from build123d import *

# Parameters (mm, degrees)
SKETCH1_W           = 115
SKETCH1_H           = 50
BOSS_EXTRUDE1_DEPTH = 29
CHAMFER1_SIZE       = 6
FILLET1_R           = 6
SKETCH2_W           = 40
SKETCH2_H           = 32
CUT_EXTRUDE1_DEPTH  = 1
CUT_EXTRUDE2_DEPTH  = 4
SKETCH4_R           = 2.031264326
CUT_EXTRUDE3_DEPTH  = 4


with BuildPart() as part:
    # Sketch1 → Boss-Extrude1 (new body)
    with BuildSketch(Plane(origin=(0, 0, 0), x_dir=(1, 0, 0), z_dir=(0, 1, 0))):
        Rectangle(SKETCH1_W, SKETCH1_H)
    extrude(amount=BOSS_EXTRUDE1_DEPTH)

    # Chamfer1
    chamfer1_edges = [part.edges().sort_by_distance(p)[0] for p in [
        (-57.5, 14.5, -25),
        (57.5, 14.5, -25),
        (57.5, 14.5, 25),
        (-57.5, 14.5, 25),
    ]]
    chamfer(chamfer1_edges, length=CHAMFER1_SIZE)

    # Fillet1
    fillet1_edges = [part.edges().sort_by_distance(p)[0] for p in [
        (0, 0, 25),
        (0, 0, -25),
        (0, 29, -25),
        (0, 29, 25),
    ]]
    fillet(fillet1_edges, radius=FILLET1_R)

    # Sketch2 → Cut-Extrude1 (cut)
    with BuildSketch(Plane(origin=(0, 29, 0), x_dir=(1, 0, 0), z_dir=(0, 1, 0))):
        with Locations((-24.5, 0)):
            Rectangle(SKETCH2_W, SKETCH2_H)
    extrude(amount=-CUT_EXTRUDE1_DEPTH, mode=Mode.SUBTRACT)

    # Sketch3 → Cut-Extrude2 (cut)
    with BuildSketch(Plane.ZY.offset(57.5)):
        with BuildLine():
            Line((-8.750173975, 13.326246728), (-4.367676958, 12.116929263))
            ThreePointArc((-4.367676958, 12.116929263), (13.18123027, 9.336320138), (-2.589295615, 17.520844884))
            Line((-2.589295615, 17.520844884), (-7.046459278, 18.931908537))
            ThreePointArc((-7.046459278, 18.931908537), (-10.774449394, 17.003213431), (-8.750173975, 13.326246728))
        make_face()
    extrude(amount=-CUT_EXTRUDE2_DEPTH, mode=Mode.SUBTRACT)

    # Sketch4 → Cut-Extrude3 (cut)
    with BuildSketch(Plane.ZY.offset(53.5)):
        with Locations((-2.116830312, 14.069543065)):
            Circle(SKETCH4_R)
    extrude(amount=-CUT_EXTRUDE3_DEPTH, mode=Mode.SUBTRACT)


solid = part.part
Work out the finished part from the listing and answer in its coordinate system (mm). A direction names the side the tool comes from. Coordinates: 2 decimals unless noted, no trailing zeros. Write each loop counter-clockwise with the first axis right and the second up, starting at its lowest first coordinate (ties: lowest second). Pieces come first, ordered by that corner, then holes.
1. For a pull along Z with two mould halves and no side action, classify faces 1 (the cylindrical face through (-55.528, 9.001, 13.064)), 2 (the flat face through (-54.5, 14.3, -22)), 3 (the cylindrical face through (-51.5, 12.8, -3.7)), 4 (the flat face through (-1, 14, 25)) as +Z half, -Z half, draft (parallel to the pull), parting line (faces both ways), or undercut.
Results list:
face 1: undercut
face 2: -Z half
face 3: undercut
face 4: +Z half
2. The part is cut by section D-D, the plane x = 7. Write down the section's boundary in (y, z), and give its area (3 significant figures).
Results list:
outline: (0, -19) arc R6 ccw to (6, -25) - (23, -25) arc R6 ccw to (29, -19) - (29, 19) arc R6 ccw to (23, 25) - (6, 25) arc R6 ccw to (0, 19) - close
area: 1,420 mm2
3. Flat-ended cylindrical pins translate along their axes: pin 1 (4.5 mm diameter, centred on y = 15, z = -2.5, fed in from -X); pin 2 (0.5 mm diameter, centred on x = -22.5, y = 28.5, fed in from -Z); pin 3 (3 mm diameter, centred on x = -26.5, y = 5, fed in from -Z); pin 4 (0.5 mm diameter, centred on x = -34, y = 28.5, fed in from +Z). Find the tip coordinate at first contact, or state that the pin passes through.
Results list:
pin 1: stops at x = -53.5
pin 2: stops at z = -21.9
pin 3: stops at z = -25
pin 4: stops at z = 21.9
4. The part is cut by section B-B, the plane y = 24.75. Write down the section's boundary in (x, z).
Results list:
outline: (-57.5, -19) - (-51.76, -24.74) - (51.76, -24.74) - (57.5, -19) - (57.5, 19) - (51.76, 24.74) - (-51.76, 24.74) - (-57.5, 19) - close
5. The part is cut by section A-A, the plane x = -21. Write down the section's boundary in (y, z).
Results list:
outline: (0, -19) arc R6 ccw to (6, -25) - (23, -25) arc R6 ccw to (29, -19) - (29, -16) - (28, -16) - (28, 16) - (29, 16) - (29, 19) arc R6 ccw to (23, 25) - (6, 25) arc R6 ccw to (0, 19) - close
6. The part is cut by section C-C, the plane z = 4.5. Write down the section's boundary in (x, y).
Results list:
outline: (-57.5, 0) - (57.5, 0) - (57.5, 29) - (-4.5, 29) - (-4.5, 28) - (-44.5, 28) - (-44.5, 29) - (-57.5, 29) - (-57.5, 21.15) - (-53.5, 21.15) - (-53.5, 3.15) - (-57.5, 3.15) - close
7. For faces 5 (the flat face through (54.5, 14.3, 22)), 6 (the flat face through (-55.528, 18.216, -4.787)), 7 (the flat face through (-25, 28, 0)), determine the directions among +Z, -Z, +X, -X, +Y, -Y from which every point of the face is accessible in a straight line to the end or side of a thin tool.
Results list:
face 5: +Z, +X, +Y, -Y
face 6: -X
face 7: +Y
8. Consider line 1 along X through (y, z) = (17.75, 2); line 2 along Y through (x, z) = (-18.5, 9); line 3 along Y through (x, z) = (17, -21). Determine where each line is inside the solid, lowest interval first.
Results list:
line 1: x = -53.5 to 57.5
line 2: y = 0 to 28
line 3: y = 0.34 to 28.66
